Geometry: final body of the model. Coordinates: model frame, mm. Give positions to 0.01 mm unless a question says otherwise; leave off trailing zeros. Loops run counter-clockwise (first coordinate to the right, second up) from the corner with the lowest first, then second, coordinate; pieces in that order, holes last. Notation, with made-up numbers: (67, 14) - (103, 14) arc R11 cw to (103, 30) - close; hole circle Ø3 at (79, -38.75). An arc over 180 degrees is marked (long way). Use one line per item in the form item = value.
```python
from build123d import *

# Parameters (mm, degrees)
SKETCH1_W           = 248
SKETCH1_H           = 78
SKETCH1_R           = 3.05
SKETCH1_W_2         = 24.2
SKETCH1_H_2         = 3.2
SKETCH1_W_3         = 3.2
SKETCH1_H_3         = 20.3
BOSS_EXTRUDE2_DEPTH = 3


with BuildPart() as part:
    # Sketch1 → Boss-Extrude2 (new body)
    with BuildSketch(Plane(origin=(0, 0, 0), x_dir=(-1, 0, 0), z_dir=(0, 0, 1))):
        with Locations((-428.787224347, 459)):
            Rectangle(SKETCH1_W, SKETCH1_H)
        with Locations(Location((-338.787224347, 436, 0), (0, 0, 180))):
            Circle(SKETCH1_R, mode=Mode.SUBTRACT)
        with Locations(Location((-368.787224347, 436, 0), (0, 0, 180))):
            Circle(SKETCH1_R, mode=Mode.SUBTRACT)
        with Locations(Location((-428.787224347, 436, 0), (0, 0, 180))):
            Circle(SKETCH1_R, mode=Mode.SUBTRACT)
        with Locations(Location((-398.787224347, 436, 0), (0, 0, 180))):
            Circle(SKETCH1_R, mode=Mode.SUBTRACT)
        with Locations(Location((-488.787224347, 436, 0), (0, 0, 180))):
            Circle(SKETCH1_R, mode=Mode.SUBTRACT)
        with Locations(Location((-458.787224347, 436, 0), (0, 0, 180))):
            Circle(SKETCH1_R, mode=Mode.SUBTRACT)
        with Locations(Location((-458.787224347, 482, 0), (0, 0, 180))):
            Circle(SKETCH1_R, mode=Mode.SUBTRACT)
        with Locations(Location((-428.787224347, 482, 0), (0, 0, 180))):
            Circle(SKETCH1_R, mode=Mode.SUBTRACT)
        with Locations(Location((-398.787224347, 482, 0), (0, 0, 180))):
            Circle(SKETCH1_R, mode=Mode.SUBTRACT)
        with Locations(Location((-368.787224347, 482, 0), (0, 0, 180))):
            Circle(SKETCH1_R, mode=Mode.SUBTRACT)
        with Locations(Location((-338.787224347, 482, 0), (0, 0, 180))):
            Circle(SKETCH1_R, mode=Mode.SUBTRACT)
        with Locations(Location((-320.787224347, 458.7, 0), (0, 0, 180))):
            Circle(SKETCH1_R, mode=Mode.SUBTRACT)
        with Locations(Location((-488.787224347, 482, 0), (0, 0, 180))):
            Circle(SKETCH1_R, mode=Mode.SUBTRACT)
        with Locations(Location((-518.787224347, 436, 0), (0, 0, 180))):
            Circle(SKETCH1_R, mode=Mode.SUBTRACT)
        with Locations(Location((-536.787224347, 459, 0), (0, 0, 180))):
            Circle(SKETCH1_R, mode=Mode.SUBTRACT)
        with Locations(Location((-518.787224347, 482, 0), (0, 0, 180))):
            Circle(SKETCH1_R, mode=Mode.SUBTRACT)
        with Locations((-383.787224347, 491.4)):
            Rectangle(SKETCH1_W_2, SKETCH1_H_2, mode=Mode.SUBTRACT)
        with Locations((-413.787224347, 491.4)):
            Rectangle(SKETCH1_W_2, SKETCH1_H_2, mode=Mode.SUBTRACT)
        with Locations((-353.787224347, 491.4)):
            Rectangle(SKETCH1_W_2, SKETCH1_H_2, mode=Mode.SUBTRACT)
        with Locations((-443.787224347, 491.4)):
            Rectangle(SKETCH1_W_2, SKETCH1_H_2, mode=Mode.SUBTRACT)
        with Locations((-473.787224347, 491.4)):
            Rectangle(SKETCH1_W_2, SKETCH1_H_2, mode=Mode.SUBTRACT)
        with Locations((-503.787224347, 491.4)):
            Rectangle(SKETCH1_W_2, SKETCH1_H_2, mode=Mode.SUBTRACT)
        with Locations((-533.787224347, 491.4)):
            Rectangle(SKETCH1_W_2, SKETCH1_H_2, mode=Mode.SUBTRACT)
        with Locations((-323.787224347, 491.4)):
            Rectangle(SKETCH1_W_2, SKETCH1_H_2, mode=Mode.SUBTRACT)
        with Locations((-313.387224347, 445.55)):
            Rectangle(SKETCH1_W_3, SKETCH1_H_3, mode=Mode.SUBTRACT)
        with Locations((-313.387224347, 471.85)):
            Rectangle(SKETCH1_W_3, SKETCH1_H_3, mode=Mode.SUBTRACT)
        with Locations((-544.187224347, 445.55)):
            Rectangle(SKETCH1_W_3, SKETCH1_H_3, mode=Mode.SUBTRACT)
        with Locations((-544.187224347, 471.85)):
            Rectangle(SKETCH1_W_3, SKETCH1_H_3, mode=Mode.SUBTRACT)
        with Locations((-533.787224347, 426)):
            Rectangle(SKETCH1_W_2, SKETCH1_H_2, mode=Mode.SUBTRACT)
        with Locations((-503.787224347, 426)):
            Rectangle(SKETCH1_W_2, SKETCH1_H_2, mode=Mode.SUBTRACT)
        with Locations((-473.787224347, 426)):
            Rectangle(SKETCH1_W_2, SKETCH1_H_2, mode=Mode.SUBTRACT)
        with Locations((-443.787224347, 426)):
            Rectangle(SKETCH1_W_2, SKETCH1_H_2, mode=Mode.SUBTRACT)
        with Locations((-413.787224347, 426)):
            Rectangle(SKETCH1_W_2, SKETCH1_H_2, mode=Mode.SUBTRACT)
        with Locations((-383.787224347, 426)):
            Rectangle(SKETCH1_W_2, SKETCH1_H_2, mode=Mode.SUBTRACT)
        with Locations((-353.787224347, 426)):
            Rectangle(SKETCH1_W_2, SKETCH1_H_2, mode=Mode.SUBTRACT)
        with Locations((-323.787224347, 426)):
            Rectangle(SKETCH1_W_2, SKETCH1_H_2, mode=Mode.SUBTRACT)
    extrude(amount=BOSS_EXTRUDE2_DEPTH)


solid = part.part
```
(1) Pin query (flat end, axial travel): P1, Ø5, axis at x = 409.5, y = -449, coming from the -Z side; P2, Ø5, axis at x = 398.79, y = -436, coming from the -Z side. Return the tip coordinate at first contact, or that it passes through.
Solution:
P1 = 0
P2 = through
(2) Pull-direction query (Y, two-part tool) for faces 1 (the face through (370.43, -433.43, 1.48)), 2 (the face through (431, -460, 0)); classes: released by +Y, released by -Y, zero draft, split by the parting line, or undercut.
Solution:
face_1 = undercut
face_2 = zero draft
(3) Cut plane A-A (x = 481.5). Return the cut outline in (y, z), plus the area to 3 significant figures.
Solution:
outline = (-498, 0) - (-493, 0) - (-493, 3) - (-498, 3) - close; (-489.8, 0) - (-427.6, 0) - (-427.6, 3) - (-489.8, 3) - close; (-424.4, 0) - (-420, 0) - (-420, 3) - (-424.4, 3) - close
area = 215 mm2
(4) Cut plane B-B (z = 1.55). Give the number of separate pieces and of enclosed holes in the cut face, plus the area to 3 significant figures.
Solution:
separate_pieces = 1
enclosed_holes = 36
area = 17,400 mm2
(5) Material intervals for L1, parallel to Y at x = 417.5, z = 0.6; L2, parallel to X at y = -474, z = 1.2; L3, parallel to X at y = -458.7, z = 0.9, sorted ascending. Write a range as from..to.
Solution:
L1 = -498..-493, -489.8..-427.6, -424.4..-420
L2 = 304.79..311.79, 314.99..542.59, 545.79..552.79
L3 = 304.79..317.74, 323.84..533.75, 539.82..552.79
